Autodesk Inventor part; units mm, degrees
ref_plane "YZ Plane" through (0, 0, 0) normal (1, 0, 0) x (0, 1, 0)
ref_plane "XZ Plane" through (0, 0, 0) normal (0, 1, 0) x (-1, 0, 0)
ref_plane "XY Plane" through (0, 0, 0) normal (0, 0, 1) x (1, 0, 0)
sketch "Sketch1" plane through (0, 0, 0) normal (0, 0, 1) x (1, 0, 0)
  line L0 (0, 0) -> (110, 0)
  line L1 (0, 42.5) -> (0, 0)
  line L2 (132, 42.5) -> (116, 42.5)
  line L3 (116, 42.5) -> (116, 46)
  line L4 (116, 46) -> (113, 46)
  line L5 (113, 46) -> (113, 42.5)
  line L6 (113, 42.5) -> (110, 42.5)
  arc A0 (110, 0) -> (132, 22) centre (110, 22) ccw
  line L7 (110, 22) -> (110, 0) construction
  line L8 (132, 22) -> (132, 42.5)
  line L9 (132, 42.5) -> (116, 42.5)
  line L10 (113, 42.5) -> (0, 42.5)
  dimension "d2" = 16
  dimension "d3" = 3.5
  dimension "thickness" = 3
  dimension "d5" = 3
  dimension "d14" = 110
  dimension "d15" = 22
  dimension "d16" = 22
  dimension "height" = 20.5
  dimension "d18" = 110
  dimension "d19" = 90
  dimension "d20" = 3
extrude "Extrusion1" add sketch "Sketch1" along normal blind 3
sketch "Sketch2" plane through (0, 0, 3) normal (0, 0, 1) x (1, 0, 0)
  line L0 (0, 42.5) -> (3, 42.5)
  line L1 (113, 42.5) -> (0, 42.5)
  line L2 (3, 42.5) -> (3, 15)
  line L3 (0, 0) -> (110, 0)
  line L4 (4, 42.5) -> (4, 15)
  line L5 (4, 42.5) -> (7, 42.5)
  line L6 (7, 42.5) -> (7, 3)
  line L7 (0, 42.5) -> (0, 0)
  line L8 (0, 0) -> (0, 15)
  line L9 (3, 15) -> (4, 15)
  line L10 (0, 42.5) -> (0, 15)
  line L11 (132, 42.5) -> (129, 42.5)
  line L12 (132, 42.5) -> (116, 42.5)
  line L13 (129, 42.5) -> (129, 22)
  arc A0 (110, 0) -> (132, 22) centre (110, 22) ccw
  line L14 (132, 22) -> (132, 42.5)
  line L15 (132, 22) -> (132, 42.5)
  line L16 (7, 0) -> (110, 0)
  line L17 (7, 3) -> (110, 3)
  line L18 (129, 22) -> (129, 22)
  arc A1 (110, 3) -> (129, 22) centre (110, 22) ccw
  arc A2 (110, 0) -> (132, 22) centre (110, 22) ccw
  line L19 (0, 0) -> (7, 0)
  dimension "d27" = 27.5
  dimension "d28" = 3
  dimension "d29" = 3
  dimension "d35" = 3
  dimension "d36" = 3
  dimension "d37" = 3
  dimension "d38" = 20.5
  dimension "d39" = 103
  dimension "d40" = 103
  dimension "d41" = 1
  dimension "d42" = 27.5
  dimension "d43" = 1
extrude "Extrusion2" add sketch "Sketch2" along normal blind 3 contours L0 L2 L9 L4 L1 L6 L17 A1 L13 L11 L14 A0 L3 L7
sketch "Sketch3" plane through (0, 0, 6) normal (0, 0, 1) x (1, 0, 0)
  line L0 (113, 42.5) -> (7, 42.5)
  line L1 (4, 42.5) -> (4, 15)
  line L2 (7, 42.5) -> (4, 42.5)
  line L3 (4, 42.5) -> (4, 15)
  line L4 (3, 42.5) -> (3, 15)
  line L5 (4, 15) -> (3, 15)
  line L6 (3, 15) -> (0, 15)
  line L7 (0, 42.5) -> (0, 0)
  line L8 (0, 15) -> (0, 0)
  line L9 (0, 0) -> (7, 0)
  line L10 (0, 0) -> (110, 0)
  arc A0 (110, 0) -> (132, 22) centre (110, 22) ccw
  line L11 (132, 22) -> (132, 42.5)
  line L12 (132, 22) -> (132, 42.5)
  line L13 (132, 42.5) -> (128.8778, 42.5)
  line L14 (132, 42.5) -> (116, 42.5)
  line L15 (7, 42.5) -> (7, 3)
  line L16 (7, 42.5) -> (7, 3)
  line L17 (110, 3) -> (7, 3)
  line L18 (7, 3) -> (110, 3)
  line L19 (129, 42.5) -> (129, 22)
  line L20 (129, 42.5) -> (129, 22)
  arc A1 (110, 3) -> (129, 22) centre (110, 22) ccw
  arc A2 (110, 0) -> (132, 22) centre (110, 22) ccw
  line L21 (7, 0) -> (110, 0)
extrude "Extrusion3" add sketch "Sketch3" along normal blind 32
sketch "Sketch5" plane through (0, 0, 38) normal (0, 0, 1) x (1, 0, 0)
  arc A0 (110, 3) -> (129, 22) centre (110, 22) ccw
  arc A1 (110, 3) -> (129, 22) centre (110, 22) ccw
  arc A2 (110, 0) -> (132, 22) centre (110, 22) ccw
  line L0 (132, 22) -> (132, 42.5)
  line L1 (132, 22) -> (132, 42.5)
  line L2 (132, 42.5) -> (129, 42.5)
  line L3 (129, 22) -> (129, 42.5)
  line L4 (129, 42.5) -> (129, 22)
  line L5 (7, 42.5) -> (7, 3)
  line L6 (110, 3) -> (7, 3)
  line L7 (7, 3) -> (7, 42.5)
  line L8 (7, 42.5) -> (4, 42.5)
  line L9 (4, 15) -> (0, 15)
  line L10 (4, 42.5) -> (4, 15)
  line L11 (3, 15) -> (3, 42.5)
  line L12 (4, 15) -> (3, 15)
  line L13 (3, 15) -> (3, 42.5)
  line L14 (113, 42.5) -> (0, 42.5)
  line L15 (3, 42.5) -> (0, 42.5)
  line L16 (0, 15) -> (0, 0)
  line L17 (0, 42.5) -> (0, 15)
  line L18 (0, 0) -> (110, 0)
  line L19 (0, 15) -> (0, 0)
  line L20 (0, 0) -> (110, 0)
  line L21 (3, 42.5) -> (0, 42.5)
  line L22 (0, 42.5) -> (0, 15)
  line L23 (3, 15) -> (3, 42.5)
  line L24 (3, 15) -> (0, 15)
  dimension "d52" = 3
extrude "Extrusion4" add sketch "Sketch5" along normal blind 3 contours A0 L3 L2 L0 A2 L18 L16 L9 L10 L8 L5 L6 | L11 L9 L17 L14
sketch "Sketch6" plane through (0, 0, 41) normal (0, 0, 1) x (1, 0, 0)
  line L0 (132, 22) -> (132, 42.5)
  line L1 (129, 22) -> (129, 42.5)
  line L2 (132, 42.5) -> (129, 42.5)
  line L3 (132, 22) -> (132, 42.5)
  line L4 (7, 42.5) -> (7, 3)
  line L5 (0, 42.5) -> (0, 0)
  line L6 (7, 42.5) -> (0, 42.5)
  line L7 (0, 42.5) -> (0, 0)
  line L8 (0, 0) -> (7, 0)
  arc A0 (110, 0) -> (132, 22) centre (110, 22) ccw
  line L9 (110, 0) -> (7, 0)
  line L10 (0, 0) -> (110, 0)
  arc A1 (110, 0) -> (132, 22) centre (110, 22) ccw
  line L11 (7, 42.5) -> (4, 42.5)
  line L12 (132, 42.5) -> (116, 42.5)
  line L13 (116, 42.5) -> (116, 46)
  line L14 (116, 42.5) -> (116, 46)
  line L15 (116, 46) -> (113, 46)
  line L16 (116, 46) -> (113, 46)
  line L17 (113, 46) -> (113, 42.5)
  line L18 (113, 46) -> (113, 42.5)
  line L19 (129, 42.5) -> (116, 42.5)
  line L20 (113, 42.5) -> (7, 42.5)
  dimension "d55" = 125
  dimension "d56" = 125
  dimension "d57" = 22
  dimension "d58" = 90
  dimension "d59" = 90
  dimension "d60" = 20.5
  dimension "d61" = 3
extrude "Extrusion5" add sketch "Sketch6" along normal blind 3
sketch "Sketch7" plane through (0, 0, 0) normal (0, -1, 0) x (1, 0, 0)
  line L0 (0, 0) -> (-15, 0)
  line L1 (0, 15) -> (0, 0)
  line L2 (0, 29) -> (0, 44)
  line L3 (-15, 15) -> (-15, 29)
  line L4 (0, 0) -> (-3, 0)
  line L5 (-12, 15) -> (-12, 29)
  line L6 (0, 0) -> (0, 6)
  line L7 (0, 0) -> (0, 3)
  line L8 (0, 44) -> (0, 41)
  line L9 (0, 38) -> (0, 44)
  arc A0 (0, 41) -> (-12, 29) centre (0, 29) ccw
  line L10 (0, 44) -> (110, 44)
  arc A1 (0, 44) -> (-15, 29) centre (0, 29) ccw
  arc A2 (-12, 15) -> (0, 3) centre (0, 15) ccw
  arc A3 (-15, 15) -> (0, 0) centre (0, 15) ccw
  dimension "d73" = 15
  dimension "d74" = 3
  dimension "d75" = 15
extrude "Extrusion6" add sketch "Sketch7" against normal blind 15
equation "\"d5\" = thickness"
equation "\"d20\" = thickness"
equation "\"d21\" = thickness"
equation "\"d28\" = thickness"
equation "\"d29\" = thickness"
equation "\"d35\" = thickness"
equation "\"d36\" = thickness"
equation "\"d37\" = thickness"
equation "\"d38\" = height"
equation "\"d44\" = thickness"
equation "\"d53\" = thickness"
equation "\"d62\" = thickness"
properties part number "boxgeneric"
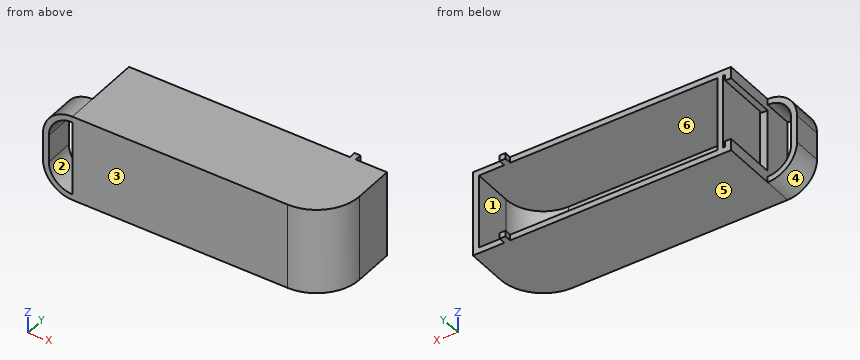
CAD build for the part. Positions are in the model's coordinates, mm. Face numbers are marked on the shaded views. A direction names the side the tool comes from. Round coordinates to 2 decimals unless told otherwise and drop trailing zeros. Write each loop counter-clockwise with the first axis right and the second up, starting at its lowest first coordinate (ties: lowest second). Pieces come first, ordered by that corner, then holes. Notation, with made-up numbers: (25, 60) - (58, 60) arc R25 ccw to (58, 72) - close; hole circle Ø3 at (-21, 5.25). An arc over 180 degrees is marked (long way). Write item = value, one per line. Start each with the question number.
Q1. Band-saw the part on C-C (x = 89). Give the cut face in (y, z), then the cut area to 3 significant figures.
Q2. Drop flat-ended pins along their axis: pin 1 (2 mm diameter, centred on x = 1, z = 23.5, fed in from +Y); pin 2 (2 mm diameter, centred on y = 24.5, z = 25, fed in from -X); pin 3 (8 mm diameter, centred on x = 57, z = 25.5, fed in from +Y). Give the stop position or say it passes through.
Q3. Band-saw the part on B-B (z = 33). Give the cut face in (x, y).
Q4. Band-saw the part on D-D (y = 10). Give the cut face in (x, z).
Q5. Mould opens along X. For the marked faces 4, 5 and 6 say: pulls with the +X half, pulls with the -X half, needs draft (parallel to the pull), parting line crosses it, or undercut.
Q6. Which spindle directions (+Z, -Z, +X, -X, +Y, -Y) get a long thin tool onto all of the face, cutting with end or side? Do the marked faces 1, 2 and 3. Say none if no direction does.
Q7. Band-saw the part on A-A (y = 30.5). Give the cut face in (x, z), then the cut area to 3 significant figures.
Q8. Probe L1, parallel to X at y = 35.5, z = 12; L2, parallel to Z at x = 28, y = 29; L3, parallel to X at y = 9.5, z = 34. List the from-to ranges inside material, lowest first. Write a range as from..to.
Answers below:
q1.outline = (0, 0) - (42.5, 0) - (42.5, 3) - (3, 3) - (3, 41) - (42.5, 41) - (42.5, 44) - (0, 44) - close
q1.area = 369 mm2
q2.pin_1 = 15
q2.pin_2 = 4
q2.pin_3 = 3
q3.outline = (-14.46, 0) - (-11.31, 0) - (-11.31, 15) - (-14.46, 15) - close; (0, 0) - (110, 0) arc R22 ccw to (132, 22) - (132, 42.5) - (129, 42.5) - (129, 22) arc R19 cw to (110, 3) - (7, 3) - (7, 42.5) - (4, 42.5) - (4, 15) - (0, 15) - close
q4.outline = (-15, 15) arc R15 ccw to (0, 0) - (128.44, 0) - (128.44, 44) - (0, 44) arc R15 ccw to (-15, 29) - close; hole (-12, 15) arc R12 ccw to (0, 3) - (0, 41) arc R12 ccw to (-12, 29) - close; hole (7, 3) - (124.73, 3) - (124.73, 41) - (7, 41) - close
q5.face_4 = pulls with the -X half
q5.face_5 = needs draft
q5.face_6 = undercut
q6.face_1 = +Y
q6.face_2 = +Y, -Y
q6.face_3 = +Z, -Z, +X, -X, -Y
q7.outline = (0, 0) - (132, 0) - (132, 44) - (0, 44) - (0, 38) - (3, 38) - (3, 41) - (4, 41) - (4, 3) - (3, 3) - (3, 6) - (0, 6) - close; hole (7, 3) - (129, 3) - (129, 41) - (7, 41) - close
q7.area = 1,040 mm2
q8.L1 = 4..7, 129..132
q8.L2 = 0..3, 41..44
q8.L3 = -14.14..-10.91, 0..7, 124.31..128.1
